```python
from build123d import *

# Parameters (mm, degrees)
M4_TAPPED_HOLE1_D     = 3.3
M4_TAPPED_HOLE1_DEPTH = 12
M4_TAPPED_HOLE1_TIP   = 0.991420021
FILLET1_R             = 0.2
CHAMFER1_SIZE         = 0.2


with BuildPart() as part:
    # Sketch1 → Revolve1 (revolve)
    with BuildSketch(Plane.XY, mode=Mode.PRIVATE) as revolve1_sk:
        Polygon((0, 0), (6, 0), (6, 11.1), (4, 11.1), (4, 27.1), (0, 27.1), align=None)
    revolve(revolve1_sk.sketch.rotate(Axis((0, 7.476190476, 0), (0, -1, 0)), 90), axis=Axis((0, 7.476190476, 0), (0, -1, 0)))

    # M4 Tapped Hole1
    with Locations(Plane(origin=(0, 0, 0), x_dir=(-1, 0, 0), z_dir=(0, -1, 0))):
        with Locations((0, 0)):
            Hole(M4_TAPPED_HOLE1_D / 2, depth=M4_TAPPED_HOLE1_DEPTH)
            with Locations((0, 0, -(M4_TAPPED_HOLE1_DEPTH + M4_TAPPED_HOLE1_TIP / 2))):  # 118° drill point
                Cone(0, M4_TAPPED_HOLE1_D / 2, M4_TAPPED_HOLE1_TIP, mode=Mode.SUBTRACT)

    # Fillet1
    fillet1_edges = [part.edges().sort_by_distance(p)[0] for p in [
        (0, 11.1, -4),
    ]]
    fillet(fillet1_edges, radius=FILLET1_R)

    # Chamfer1
    chamfer1_edges = [part.edges().sort_by_distance(p)[0] for p in [
        (0, 27.1, -4),
        (0, 11.1, -6),
        (0, 0, -6),
    ]]
    chamfer(chamfer1_edges, length=CHAMFER1_SIZE)


solid = part.part
```
Geometry check sheet. Reference: the model listing, model coordinates, mm. A direction names the side the tool comes from. Coordinates: 2 decimals unless noted, no trailing zeros. Order: outer loops, then holes, each group sorted by start corner. A loop starts at its lowest first (then second) coordinate and runs counter-clockwise, first axis right, second up.
Item 1: Mould release check, pull along Z, two halves, no side actions. Record for faces 3 (the flat face through (-1.4, 0, -1.2)), 4 (the cylindrical face through (-1.216, 6.084, -1.115)), 5 (the cylindrical face through (3.905, 19.209, -0.867)): released by +Z, released by -Z, zero draft, split by the parting line, or undercut.
Item 2: Section check B-B (y = 18). Enter the section's corners in (x, z), plus the area to 3 significant figures.
Item 3: Section check A-A (y = 9). Enter the section's corners in (x, z).
Item 4: Depth check by flat-ended pin: pin 1 (5 mm diameter, centred on x = 1, y = 21.5, fed in from -Z); pin 2 (1.5 mm diameter, centred on y = 3.5, z = 4.5, fed in from +X); pin 3 (6 mm diameter, centred on y = 22.5, z = 1, fed in from +X). Enter the tip coordinate at first touch or a pass-through.
Item 5: Tool access check on faces 1 (the conical face through (0.1, 12.8, 0.3)), 2 (the flat face through (-2, 11.1, 4)). Record the directions out of +Z, -Z, +X, -X, +Y, -Y that give a thin tool (end or side, any length) a straight path to the whole face; none if there is none.
Item 6: Scan lines: line 1 along Y through (x, z) = (3.75, -4); line 2 along X through (y, z) = (2.5, 1.25); line 3 along Z through (x, y) = (3.5, 17.25). Record each from-to range of solid material in increasing order.
Check sheet entries:
1. face 3: zero draft
1. face 4: undercut
1. face 5: split by the parting line
2. outline: circle Ø8 at (0, 0)
2. area: 50.3 mm2
3. outline: circle Ø12 at (0, 0); hole circle Ø3.3 at (0, 0)
4. pin 1: stops at z = -4
4. pin 2: stops at x = 4.68
4. pin 3: stops at x = 4
5. face 1: -Y
5. face 2: +Y
6. line 1: y = 0 to 11.1
6. line 2: x = -5.87 to -1.08, 1.08 to 5.87
6. line 3: z = -1.94 to 1.94
